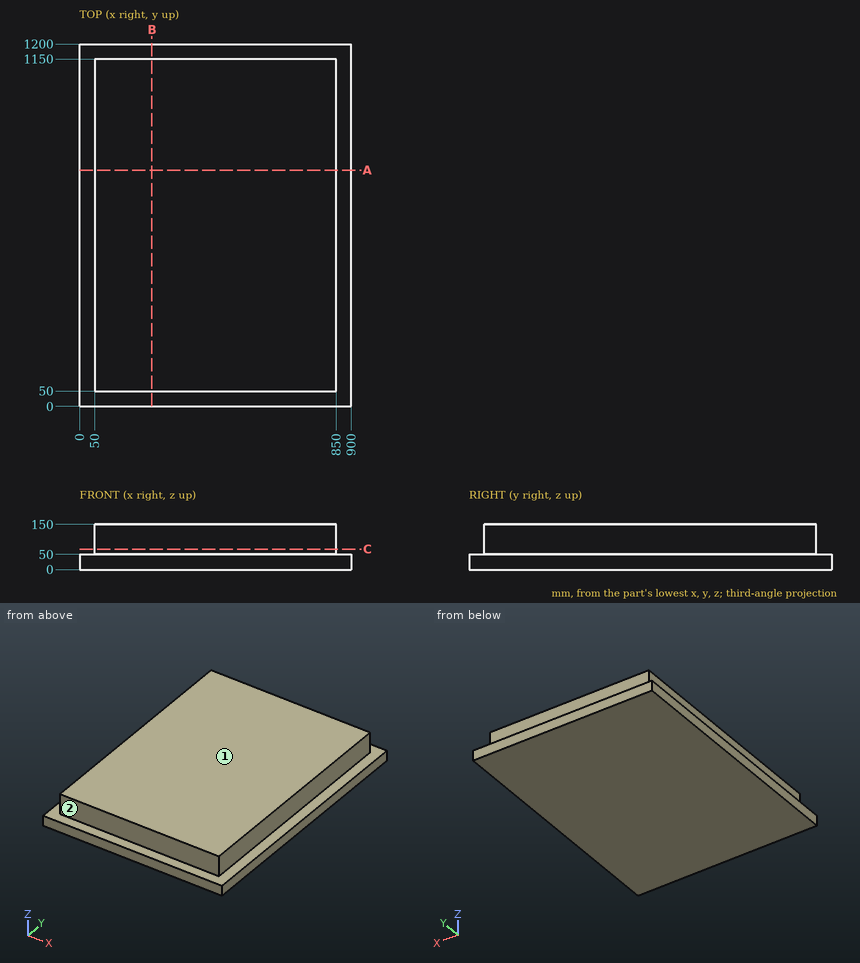
Print and shaded views of the part. All mm, measured from the part's lowest x, y and z. A direction names the side the tool comes from. Give positions to 0.01 mm unless a question says otherwise; leave off trailing zeros. Loops run counter-clockwise (first coordinate to the right, second up) from the corner with the lowest first, then second, coordinate; pieces in that order, holes last. Notation, with made-up numbers: (22.25, 3) - (80.25, 3) arc R25 ccw to (80.25, 32) - close; hole circle Ø1 at (3, 66). An arc over 180 degrees is marked (long way). One line per item, written item: value. Start each with the question number.
1. Slice it at A-A (y = 782). List the corners of the cut face in (x, z).
2. Pin check, flat tips, straight feed: pin 1 (1 mm diameter, centred on x = 577.5, y = 629.5, fed in from -Z); pin 2 (2 mm diameter, centred on y = 134.5, z = 85, fed in from +X); pin 3 (5 mm diameter, centred on y = 839.5, z = 66.5, fed in from -X). Stop position of each tip, or through.
3. Probe L1, parallel to Y at x = 328, z = 71; L2, parallel to X at y = 64.5, z = 126.5. List the from-to ranges inside material, lowest first. Write a range as from..to.
4. Slice it at C-C (z = 68). List the corners of the cut face in (x, y), plus the area to 3 significant figures.
5. Which spindle directions (+Z, -Z, +X, -X, +Y, -Y) get a long thin tool onto all of the face, cutting with end or side? Do the marked faces 1 and 2. Say none if no direction does.
6. Slice it at B-B (x = 239.5). List the corners of the cut face in (y, z).
Solution:
1. outline: (0, 0) - (900, 0) - (900, 50) - (850, 50) - (850, 150) - (50, 150) - (50, 50) - (0, 50) - close
2. pin 1: stops at z = 0
2. pin 2: stops at x = 850
2. pin 3: stops at x = 50
3. L1: y = 50..1150
3. L2: x = 50..850
4. outline: (50, 50) - (850, 50) - (850, 1150) - (50, 1150) - close
4. area: 880,000 mm^2
5. face 1: +Z, +X, -X, +Y, -Y
5. face 2: +Z, +X, -X, -Y
6. outline: (0, 0) - (1200, 0) - (1200, 50) - (1150, 50) - (1150, 150) - (50, 150) - (50, 50) - (0, 50) - close
